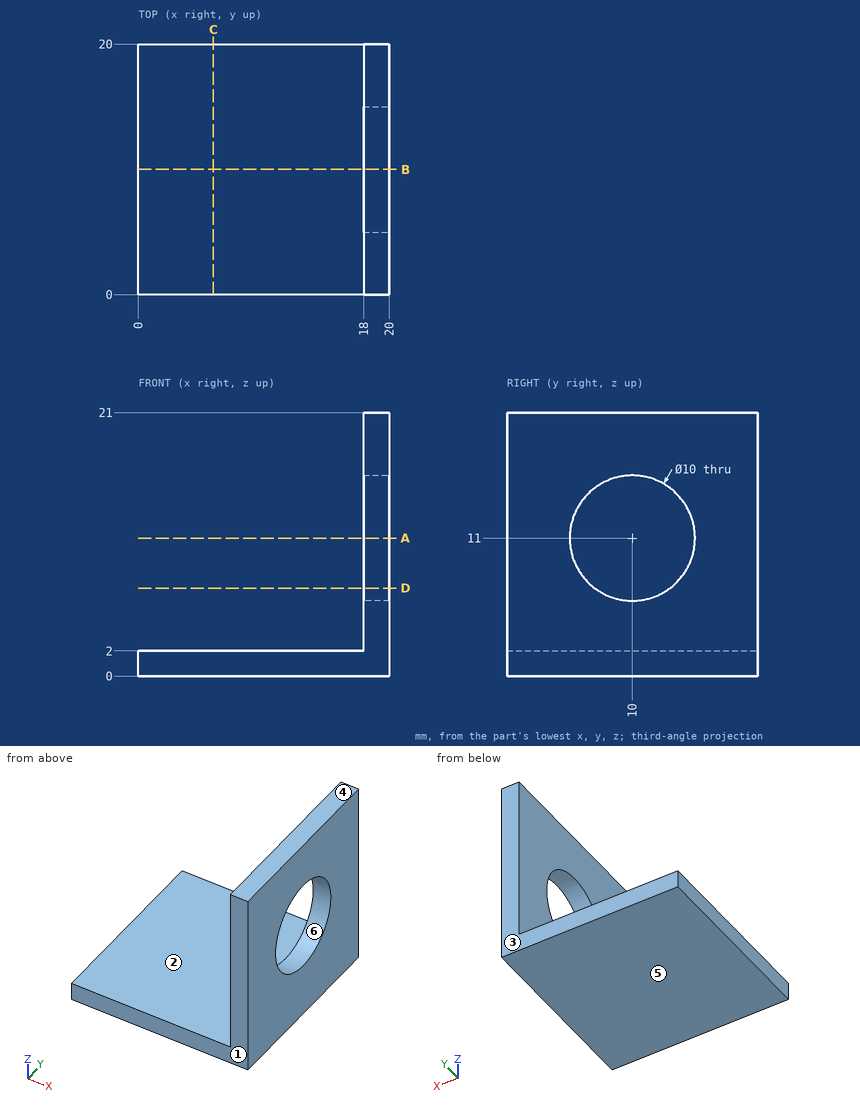
Study the drawing (mm; zero at the part's minimum x, y, z) and answer. A direction names the side the tool comes from. Give positions to 0.01 mm unless a question says otherwise; leave off trailing zeros. Order: outer loops, then holes, each group sorted by start corner. A loop starts at its lowest first (then second) coordinate and runs counter-clockwise, first axis right, second up. Notation, with made-up numbers: M 50.25,16 L 81.25,16 A20 ccw 81.25,26 Z; hole C -18.75,-6.5 d5. An arc over 180 degrees is marked long. Put each result on its own line as item: value. Start each with the question number.
Item 1: Which of the six approach directions +Z, -Z, +X, -X, +Y, -Y give full straight-line access (tool end or side, diameter ignored) to the marked faces 1 and 2?
Item 2: Find the intervals of material crossed by line 1 along Y through (x, z) = (19.2, 11); line 2 along Z through (x, y) = (10.5, 2); line 3 along X through (y, z) = (16, 18.25), in increasing order.
Item 3: For a pull along Z with two mould halves and no side action, classify the marked faces 3, 4, 5 and 6 as +Z half, -Z half, draft (parallel to the pull), parting line (faces both ways), or undercut.
Item 4: The part is cut by section C-C, the plane x = 6. Determine the outline of the cut face in (y, z).
Item 5: The part is cut by section A-A, the plane z = 11. Determine the outline of the cut face in (x, y).
Item 6: Flat-ended cylindrical pins translate along their axes: P1, Ø6, axis at x = 8, y = 3, coming from the -Z side; P2, Ø9, axis at x = 7, y = 12.5, coming from the +Z side; P3, Ø6, axis at y = 10, z = 11, coming from the -X side; P4, Ø9.5, axis at y = 9, z = 14, coming from the -X side. Find the tip coordinate at first contact, or state that the pin passes through.
Item 7: The part is cut by section D-D, the plane z = 7. Determine the outline of the cut face in (x, y).
Item 8: The part is cut by section B-B, the plane y = 10. Determine the outline of the cut face in (x, z).
Answer key:
1. face 1: +Z, -Z, +X, -X, -Y
1. face 2: +Z, -X, +Y, -Y
2. line 1: y = 0 to 5, 15 to 20
2. line 2: z = 0 to 2
2. line 3: x = 18 to 20
3. face 3: draft
3. face 4: +Z half
3. face 5: -Z half
3. face 6: undercut
4. outline: M 0,0 L 20,0 L 20,2 L 0,2 Z
5. outline: M 18,0 L 20,0 L 20,5 L 18,5 Z; M 18,15 L 20,15 L 20,20 L 18,20 Z
6. P1: stops at z = 0
6. P2: stops at z = 2
6. P3: passes through
6. P4: stops at x = 18
7. outline: M 18,0 L 20,0 L 20,7 L 18,7 Z; M 18,13 L 20,13 L 20,20 L 18,20 Z
8. outline: M 0,0 L 20,0 L 20,6 L 18,6 L 18,2 L 0,2 Z; M 18,16 L 20,16 L 20,21 L 18,21 Z
